```python
from build123d import *

# Parameters (mm, degrees)
F0_W     = 76.2
F0_H     = 152.4
F1_DEPTH = 12.7
F2_T     = -2.54
F4_DEPTH = 58.25523
F5_R     = 5.08


with BuildPart() as f1:
    # F0 (on Top) → F1 (new body)
    with BuildSketch(Plane.XY):
        with Locations((-4.155798, -0.207823)):
            Rectangle(F0_W, F0_H)
    extrude(amount=-F1_DEPTH)

    # F2
    f2_openings = [f1.faces().sort_by_distance(p)[0] for p in [
        (-4.155798, -0.207823, 0),
    ]]
    offset(amount=F2_T, openings=f2_openings)

    # F3 (on face) → F4 (cut)
    with BuildSketch(Plane.XY.offset(-10.16)):
        Polygon((-35.365767, 48.259617), (-25.284341, 43.805525), (-15.516325, 48.91042), (-13.417234, 59.730213), (-20.567727, 68.117378), (-31.583337, 67.75621), (-38.169084, 58.918675), align=None)
    extrude(amount=-F4_DEPTH, mode=Mode.SUBTRACT)

    # F5
    f5_edges = [f1.edges().sort_by_distance(p)[0] for p in [
        (33.944202, -76.407823, -6.35),
        (-42.255798, -76.407823, -6.35),
        (33.944202, 75.992177, -6.35),
        (-42.255798, 75.992177, -6.35),
    ]]
    fillet(f5_edges, radius=F5_R)


solid = f1.part
```
Verification items for the finished model (mm, model axes). A direction names the side the tool comes from. Give positions to 0.01 mm unless a question says otherwise; leave off trailing zeros. Order: outer loops, then holes, each group sorted by start corner. A loop starts at its lowest first (then second) coordinate and runs counter-clockwise, first axis right, second up. Notation, with made-up numbers: M 43,29.5 L 70,29.5 A22 ccw 70,67.5 Z; hole C 46,27 d3. An arc over 180 degrees is marked long. Return JSON: item names as keys, results as strings. Group by question number.
1) Section check A-A on x = 5. Record the cut outline in (y, z).
2) Mould release check, pull along X, two halves, no side actions. Record for faces 4 (the face through (32, 23, 0)), 5 (the face through (-5, 73.452, -5)), 6 (the face through (33.944, -1, -6)): pulls with the +X half, pulls with the -X half, needs draft (parallel to the pull), parting line crosses it, or undercut.
3) Section check B-B on y = 56.5. Record the cut outline in (x, z).
4) Go/stop test with a flat-tipped pin: pin 1 Ø8 at (x, y) = (-28.5, -7) entering from +Z. Record where the tip stops, or that it passes through.
5) Scan lines: line 1 (X direction, y = -30.5, z = -4.25); line 2 (Y direction, x = -4, z = -4); line 3 (Z direction, x = -8, y = -3). Record each from-to range of solid material in increasing order.
6) Section check D-D on x = -30. Record the cut outline in (y, z).
7) Access from +Z, -Z, +X, -X, +Y, -Y to the whole of each face (thin tool, end or side, straight path). Record for faces 1 (the face through (-36.787, 53.664, -11.412)), 2 (the face through (-5, 1, -12.7)), 3 (the face through (31.404, -1, -5)).
8) Section check C-C on z = -1.75. Record the cut outline in (x, y).
Answer block:
{
 "1": {"outline": "M -76.41,-12.7 L 75.99,-12.7 L 75.99,0 L 73.45,0 L 73.45,-10.16 L -73.87,-10.16 L -73.87,0 L -76.41,0 Z"},
 "2": {"face 4": "needs draft", "face 5": "undercut", "face 6": "pulls with the +X half"},
 "3": {"outline": "M -42.26,-12.7 L -37.53,-12.7 L -37.53,-10.16 L -39.72,-10.16 L -39.72,0 L -42.26,0 Z; M -14.04,-12.7 L 33.94,-12.7 L 33.94,0 L 31.4,0 L 31.4,-10.16 L -14.04,-10.16 Z"},
 "4": {"pin 1": "stops at z = -10.16"},
 "5": {"line 1": "x = -42.26 to -39.72, 31.4 to 33.94", "line 2": "y = -76.41 to -73.87, 73.45 to 75.99", "line 3": "z = -12.7 to -10.16"},
 "6": {"outline": "M -76.41,-12.7 L 45.89,-12.7 L 45.89,-10.16 L -73.87,-10.16 L -73.87,0 L -76.41,0 Z; M 67.81,-12.7 L 75.99,-12.7 L 75.99,0 L 73.45,0 L 73.45,-10.16 L 67.81,-10.16 Z"},
 "7": {"face 1": "+Z, -Z", "face 2": "-Z, +X, -X, +Y, -Y", "face 3": "+Z"},
 "8": {"outline": "M -42.26,-71.33 A5.08 ccw -37.18,-76.41 L 28.86,-76.41 A5.08 ccw 33.94,-71.33 L 33.94,70.91 A5.08 ccw 28.86,75.99 L -37.18,75.99 A5.08 ccw -42.26,70.91 Z; hole M -39.72,-73.87 L 31.4,-73.87 L 31.4,73.45 L -39.72,73.45 Z"}
}
